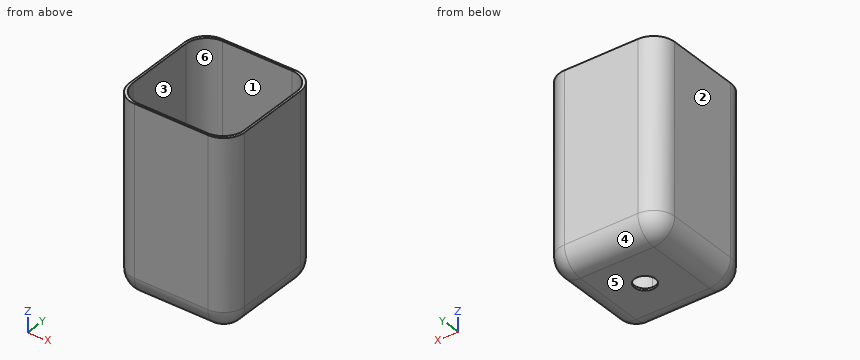
Autodesk Fusion 360 part; units mm, degrees
sketch "Esquisse1" plane through (0, 0, 0) normal (0, 0, 1) x (1, 0, 0)
  line L0 (0, 0) -> (53, 0)
  line L1 (53, 0) -> (53, 53)
  line L2 (53, 53) -> (0, 53)
  line L3 (0, 53) -> (0, 0)
  line L4 (54, -1) -> (54, 54)
  line L5 (54, 54) -> (-1, 54)
  line L6 (-1, 54) -> (-1, -1)
  line L7 (-1, -1) -> (54, -1)
  line L8 (26.5, 53) -> (26.5, 0)
  circle A0 centre (26.5, 26.5) radius 5
  dimension "d4" = 53
  dimension "d5" = 53
  dimension "d6" = 1
  dimension "d20" = 10
extrude "Extrusion1" add sketch "Esquisse1" along normal blind 90
extrude "Extrusion2" add sketch "Esquisse1" along normal blind 1 contours L0 L2 L3 L8 A0 | L0 L1 L2 L8 A0 | L8 A0 | L8 A0
fillet "Congé1" radius 10 4 edges at (0, 53, 45.5) (53, 53, 45.5) (53, 0, 45.5) (0, 0, 45.5)
fillet "Congé2" radius 10 8 edges at (50.0711, 50.0711, 1) (53, 26.5, 1) (50.0711, 2.9289, 1) (26.5, 0, 1) (2.9289, 2.9289, 1) (0, 26.5, 1) (2.9289, 50.0711, 1) (26.5, 53, 1)
fillet "Congé3" radius 10 4 edges at (-1, 54, 45) (54, 54, 45) (54, -1, 45) (-1, -1, 45)
fillet "Congé4" radius 10 8 edges at (54, 26.5, 0) (51.0711, 51.0711, 0) (26.5, 54, 0) (1.9289, 51.0711, 0) (-1, 26.5, 0) (1.9289, 1.9289, 0) (26.5, -1, 0) (51.0711, 1.9289, 0)
extrude "Extrusion3" cut sketch "Esquisse1" along normal blind 1 contours L8 A0 | L8 A0
equation "base_largeur = 53 mm"
equation "epaisseur = 1 mm"
equation "hauteur = 90 mm"
equation "d4 = base_largeur"
equation "d5 = base_largeur"
equation "d6 = epaisseur"
equation "d7 = hauteur"
equation "d9 = epaisseur"
equation "angle_int = 10 mm"
equation "d13 = angle_int"
equation "d15 = angle_int"
equation "d17 = angle_int"
equation "d19 = angle_int"
equation "d21 = epaisseur"
Source: CAD feature listing. Evaluate the final solid. Frame: model axes, mm. Face numbers are marked on the shaded views. A direction names the side the tool comes from. Give positions to 0.01 mm unless a question says otherwise; leave off trailing zeros. Write each loop counter-clockwise with the first axis right and the second up, starting at its lowest first coordinate (ties: lowest second). Pieces come first, ordered by that corner, then holes.
1. Material intervals for line 1 along X through (y, z) = (32, 80); line 2 along Z through (x, y) = (37.5, 39.5), sorted ascending.
2. Section query D-D (y = 19). Return the cut outline in (x, z).
3. Access query for the marked faces 1 and 2. Directions: +Z, -Z, +X, -X, +Y, -Y. A direction counts if a zero-diameter tool reaches every point of the face in a straight line with its end or side. Return the directions, or none.
4. Section query A-A (x = 26.5). Return the cut outline in (y, z).
5. Pull-direction query (Y, two-part tool) for the marked faces 3, 4, 5 and 6; classes: +Y half, -Y half, draft (parallel to the pull), parting line (faces both ways), or undercut.
6. Section query C-C (z = 41.5). Return the cut outline in (x, y), then the cut area to 3 significant figures.
Output values:
1. line 1: x = -1 to 0, 53 to 54
1. line 2: z = 0 to 1
2. outline: (-1, 10) arc R10 ccw to (9, 0) - (44, 0) arc R10 ccw to (54, 10) - (54, 90) - (53, 90) - (53, 11) arc R10 cw to (43, 1) - (10, 1) arc R10 cw to (0, 11) - (0, 90) - (-1, 90) - close
3. face 1: +Z
3. face 2: +Z, -Z, -X, +Y, -Y
4. outline: (-1, 10) arc R10 ccw to (9, 0) - (21.5, 0) - (21.5, 1) - (10, 1) arc R10 cw to (0, 11) - (0, 90) - (-1, 90) - close; (31.5, 0) - (44, 0) arc R10 ccw to (54, 10) - (54, 90) - (53, 90) - (53, 11) arc R10 cw to (43, 1) - (31.5, 1) - close
5. face 3: undercut
5. face 4: +Y half
5. face 5: draft
5. face 6: undercut
6. outline: (-1, 9) arc R10 ccw to (9, -1) - (44, -1) arc R10 ccw to (54, 9) - (54, 44) arc R10 ccw to (44, 54) - (9, 54) arc R10 ccw to (-1, 44) - close; hole (0, 10) arc R10 ccw to (10, 0) - (43, 0) arc R10 ccw to (53, 10) - (53, 43) arc R10 ccw to (43, 53) - (10, 53) arc R10 ccw to (0, 43) - close
6. area: 216 mm2
